Autodesk Inventor part; units mm, degrees
ref_plane "YZ Plane" through (0, 0, 0) normal (1, 0, 0) x (0, 1, 0)
ref_plane "XZ Plane" through (0, 0, 0) normal (0, 1, 0) x (-1, 0, 0)
ref_plane "XY Plane" through (0, 0, 0) normal (0, 0, 1) x (1, 0, 0)
sketch "草图1" plane through (0, 0, 0) normal (0, 1, 0) x (-1, 0, 0)
  line L0 (0, 0) -> (50, 0)
  line L1 (50, 0) -> (50, -20)
  line L2 (50, -20) -> (0, -20)
  line L3 (0, -20) -> (0, 0)
  line L4 (35, -20) -> (15, -20)
  line L5 (15, -20) -> (15, -70)
  line L6 (15, -70) -> (35, -70)
  line L7 (35, -70) -> (35, -20)
  line L8 (25, 0) -> (25, -7.1636)
  line L9 (50, -20) -> (35, -70)
  line L10 (15, -70) -> (0, -20)
  circle A0 centre (40, -10) radius 2.55
  circle A1 centre (10, -10) radius 2.55
  circle A2 centre (25, -30) radius 2.55
  circle A3 centre (25, -60) radius 2.55
  line L11 (50, -10) -> (45.4992, -10)
  dimension "d0" = 50
  dimension "d1" = 20
  dimension "d2" = 20
  dimension "d3" = 50
  dimension "d4" = 5.1
  dimension "d5" = 10
  dimension "d6" = 10
  dimension "d7" = 10
extrude "拉伸1" add sketch "草图1" along normal blind 3
chamfer "倒角1" distance 4 angle 45 2 edges at (0, 1.5, 0) (-50, 1.5, 0)
chamfer "倒角2" distance 4 angle 45 2 edges at (-15, 1.5, -70) (-35, 1.5, -70)
properties part number "body_fix2"
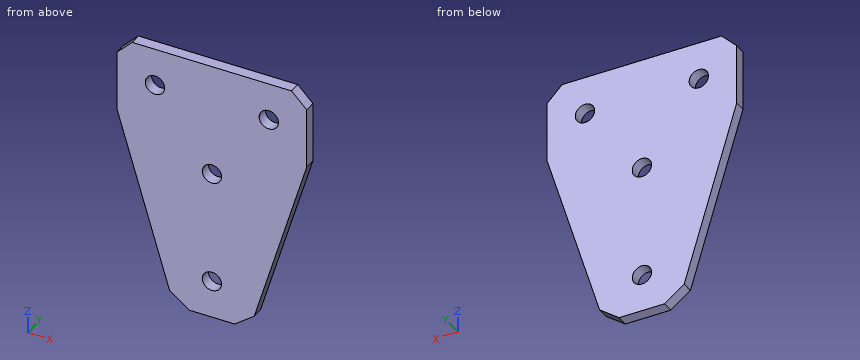
For this review, take the finished solid that the model builds, in its own axes (mm). Coordinates: 2 decimals unless noted, no trailing zeros. Order: outer loops, then holes, each group sorted by start corner. A loop starts at its lowest first (then second) coordinate and runs counter-clockwise, first axis right, second up. Notation, with made-up numbers: (9, 2) - (52, 2) arc R23 cw to (52, 34) - close; hole circle Ø4 at (17.25, 73.5). An arc over 180 degrees is marked (long way). Answer as a JSON object with one key per item and string values. Group by question number.
1. We need section C-C on y = 1.8. State the section outline as (x, z) points, then the cut area to 3 significant figures.
2. We need section D-D on z = -60. State the section outline as (x, y) points, then the cut area to 3 significant figures.
3. Clearance check with a flat-ended pin moving along its axis: P1, Ø1.5, axis at x = -34, z = -7.5, coming from the -Y side. State where the tip first meets the part, or that it passes through.
4. For probe 1 along Z at (x, y) = (-25, 1); probe 2 along Z at (x, y) = (-26, 1.1); probe 3 along X at (y, z) = (1.5, -55.5), list the stretches that pass through material, from the lowest coordinate up.
5. We need section B-B on z = -10. State the section outline as (x, y) points, then the cut area to 3 significant figures.
6. We need section A-A on x = -25. State the section outline as (y, z) points.
Final values:
{
 "1": {"outline": "(-50, -20) - (-36.15, -66.17) - (-31, -70) - (-19, -70) - (-13.85, -66.17) - (0, -20) - (0, -4) - (-4, 0) - (-46, 0) - (-50, -4) - close; hole circle Ø5.1 at (-40, -10); hole circle Ø5.1 at (-25, -60); hole circle Ø5.1 at (-25, -30); hole circle Ø5.1 at (-10, -10)", "area": "2,640 mm²"},
 "2": {"outline": "(-38, 0) - (-27.55, 0) - (-27.55, 3) - (-38, 3) - close; (-22.45, 0) - (-12, 0) - (-12, 3) - (-22.45, 3) - close", "area": "62.7 mm²"},
 "3": {"P1": "y = 0"},
 "4": {"probe 1": "-70 to -62.55, -57.45 to -32.55, -27.45 to 0", "probe 2": "-70 to -62.35, -57.65 to -32.35, -27.65 to 0", "probe 3": "-39.35 to -10.65"},
 "5": {"outline": "(-50, 0) - (-42.55, 0) - (-42.55, 3) - (-50, 3) - close; (-37.45, 0) - (-12.55, 0) - (-12.55, 3) - (-37.45, 3) - close; (-7.45, 0) - (0, 0) - (0, 3) - (-7.45, 3) - close", "area": "119 mm²"},
 "6": {"outline": "(0, -70) - (3, -70) - (3, -62.55) - (0, -62.55) - close; (0, -57.45) - (3, -57.45) - (3, -32.55) - (0, -32.55) - close; (0, -27.45) - (3, -27.45) - (3, 0) - (0, 0) - close"}
}
